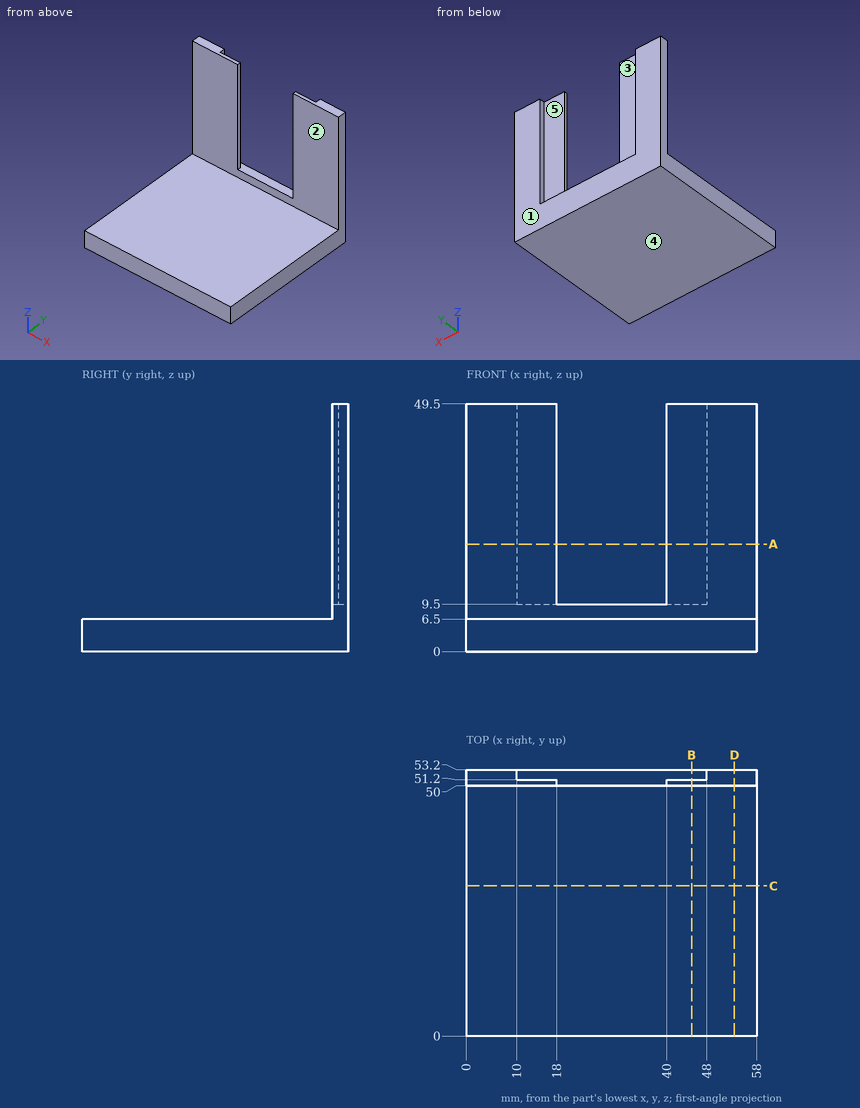
Can you work these out from the drawing? Everything is in mm from the part's minimum corner. A direction names the side the tool comes from. Round coordinates to 2 decimals unless told otherwise and drop trailing zeros. Loops run counter-clockwise (first coordinate to the right, second up) from the corner with the lowest first, then second, coordinate; pieces in that order, holes last. Notation, with made-up numbers: (38.25, -22.5) -> (47.25, -22.5) arc R25 cw to (47.25, 0.5) -> close; hole circle Ø10 at (-28, -7.75). An arc over 180 degrees is marked (long way). Use CSV: the item, a comma, the result in double quotes.
(1) If I drill on probe 1 along Z at (x, y) = (10, 28.5); probe 2 along Y at (x, z) = (55, 38); probe 3 along Y at (x, z) = (44.5, 28.5), over which ranges is the centre line in solid material (lowest first)? Write a range as [from, to].
Return value:
probe 1,"z = [0, 6.5]"
probe 2,"y = [50, 53.2]"
probe 3,"y = [50, 51.2]"
(2) Suppose I cut it at B-B on x = 45. Write out the boundary of the cut face in (y, z), plus the area to 3 significant figures.
Return value:
outline,"(0, 0) -> (53.2, 0) -> (53.2, 9.5) -> (51.2, 9.5) -> (51.2, 49.5) -> (50, 49.5) -> (50, 6.5) -> (0, 6.5) -> close"
area,"403 mm²"
(3) Suppose I cut it at A-A on z = 21.5. Write out the boundary of the cut face in (x, y), plus the area to 3 significant figures.
Return value:
outline,"(0, 50) -> (18, 50) -> (18, 51.2) -> (10, 51.2) -> (10, 53.2) -> (0, 53.2) -> close; (40, 50) -> (58, 50) -> (58, 53.2) -> (48, 53.2) -> (48, 51.2) -> (40, 51.2) -> close"
area,"83.2 mm²"
(4) If we mould it in two halves opening along X, with no side actions, what happens to the marked faces 4 and 5? For each: +X half, -X half, draft (parallel to the pull), parting line (faces both ways), or undercut.
Return value:
face 4,"draft"
face 5,"undercut"
(5) Will these pins go through, and if not, where does the flat tip stop? pin 1 Ø2 at (x, y) = (41.5, 30.5) entering from +Z; pin 2 Ø6.5 at (x, z) = (13.5, 35) entering from +Y; pin 3 Ø2.5 at (x, y) = (32.5, 51.5) entering from +Z.
Return value:
pin 1,"stops at z = 6.5"
pin 2,"stops at y = 51.2"
pin 3,"stops at z = 9.5"
(6) For the marked faces 1, 2 and 3, which set-ups out of +Z, -Z, +X, -X, +Y, -Y let a thin tool reach every point of the face, with its end or its side?
Return value:
face 1,"+Z, -Z, +X, -X, +Y"
face 2,"+Z, +X, -X, -Y"
face 3,"+Z, +Y"
(7) Suppose I cut it at C-C on y = 30. Write out the boundary of the cut face in (x, z), plus the area to 3 significant figures.
Return value:
outline,"(0, 0) -> (58, 0) -> (58, 6.5) -> (0, 6.5) -> close"
area,"377 mm²"
(8) Suppose I cut it at D-D on x = 53.5. Write out the boundary of the cut face in (y, z), plus the area to 3 significant figures.
Return value:
outline,"(0, 0) -> (53.2, 0) -> (53.2, 49.5) -> (50, 49.5) -> (50, 6.5) -> (0, 6.5) -> close"
area,"483 mm²"
